```python
from build123d import *

# Parameters (mm, degrees)
EXTRUDE_THIN1_DEPTH = 9.75
SKETCH3_W           = 15
SKETCH3_H           = 9.75
BOSS_EXTRUDE1_DEPTH = 2
SKETCH4_R           = 2.25
CUT_EXTRUDE1_DEPTH  = 25.188065239


with BuildPart() as part:
    # Sketch1 → Extrude-Thin1 (new body)
    with BuildSketch(Plane.XY):
        with BuildLine():
            ThreePointArc((-6, 0), (0, -6), (6, 0))
            Line((6, 0), (7, 0))
            ThreePointArc((7, 0), (0, -7), (-7, 0))
            Line((-7, 0), (-6, 0))
        make_face()
    extrude(amount=EXTRUDE_THIN1_DEPTH)

    # Sketch3 → Boss-Extrude1 (add)
    with BuildSketch(Plane(origin=(0, 0, 0), x_dir=(1, 0, 0), z_dir=(0, 1, 0))):
        with Locations((-13.5, -4.875)):
            Rectangle(SKETCH3_W, SKETCH3_H)
        with Locations((13.5, -4.875)):
            Rectangle(SKETCH3_W, SKETCH3_H)
    extrude(amount=-BOSS_EXTRUDE1_DEPTH)

    # Sketch4 → Cut-Extrude1 (cut, through all)
    with BuildSketch(Plane(origin=(0, 0, 0), x_dir=(1, 0, 0), z_dir=(0, 1, 0))):
        with Locations(Location((-17, -4.875, 0), (0, 0, 180))):
            Circle(SKETCH4_R)
        with Locations((17, -4.875)):
            Circle(SKETCH4_R)
    extrude(amount=-CUT_EXTRUDE1_DEPTH, mode=Mode.SUBTRACT)


solid = part.part
```
CAD build for the part. Positions are in the model's coordinates, mm. A direction names the side the tool comes from. Give positions to 0.01 mm unless a question says otherwise; leave off trailing zeros. Order: outer loops, then holes, each group sorted by start corner. A loop starts at its lowest first (then second) coordinate and runs counter-clockwise, first axis right, second up. Notation, with made-up numbers: M -35.5,40 L 13.5,40 A11 ccw 13.5,44 Z; hole C -10,45.25 d11. An arc over 180 degrees is marked long. Put each result on its own line as item: value. Start each with the question number.
(1) Drill centre lines: line 1 along Z through (x, y) = (-17, -1.35) (3 decimals); line 2 along Y through (x, z) = (-14, 7.75); line 3 along X through (y, z) = (-1.5, 4.75). Where is each one in solid material? Low to high.
(2) Saw through at A-A, the plane x = -17. Write the cut outline in (y, z) (3 decimals).
(3) Saw through at C-C, the plane y = -5. Write the cut outline in (x, z).
(4) Saw through at B-B, the plane z = 6. Write the cut outline in (x, y), then the cut area to 3 significant figures.
(5) Flat gauge pins, fed straight in: pin 1 Ø5 at (x, z) = (-17, 4.875) entering from -Y; pin 2 Ø4 at (y, z) = (-4.5, 1.5) entering from -X; pin 3 Ø4 at (x, z) = (-6, 7) entering from -Y. Where does each tip first touch, or does it go through?
(6) Mould opens along X. For faces 3 (the flat face through (21, -1, 5)), 4 (the cylindrical face through (0, -6, 5)), 5 (the flat face through (-14, -2, 5)) say: +X half, -X half, draft (parallel to the pull), parting line (faces both ways), or undercut.
(7) Saw through at D-D, the plane z = 8.5. Write the cut outline in (x, y), then the cut area to 3 significant figures.
(8) Which spindle directions (+Z, -Z, +X, -X, +Y, -Y) get a long thin tool onto all of the face, cutting with end or side? Do faces 1 (the cylindrical face through (-19.146, -0.986, 5.551)), 2 (the flat face through (14, -2, 5)). Say none if no direction does.
Check result:
1. line 1: z = 0 to 2.625, 7.125 to 9.75
1. line 2: y = -2 to 0
1. line 3: x = -21 to -19.25, -14.75 to -5.81, 5.81 to 14.75, 19.25 to 21
2. outline: M -2,0 L 0,0 L 0,2.625 L -2,2.625 Z; M -2,7.125 L 0,7.125 L 0,9.75 L -2,9.75 Z
3. outline: M -4.9,0 L -3.32,0 L -3.32,9.75 L -4.9,9.75 Z; M 3.32,0 L 4.9,0 L 4.9,9.75 L 3.32,9.75 Z
4. outline: M -21,-2 L -18.95,-2 L -18.95,0 L -21,0 Z; M -15.05,-2 L -6.71,-2 A7 ccw 6.71,-2 L 15.05,-2 L 15.05,0 L 6,0 A6 cw -6,0 L -15.05,0 Z; M 18.95,-2 L 21,-2 L 21,0 L 18.95,0 Z
4. area: 61.2 mm2
5. pin 1: stops at y = -2
5. pin 2: stops at x = -6.54
5. pin 3: stops at y = -5.74
6. face 3: +X half
6. face 4: undercut
6. face 5: draft
7. outline: M -21,-2 L -6.71,-2 A7 ccw 6.71,-2 L 21,-2 L 21,0 L 6,0 A6 cw -6,0 L -21,0 Z
7. area: 76.8 mm2
8. face 1: +Y, -Y
8. face 2: +Z, -Z, +X, -Y
